from build123d import *

# Parameters (mm, degrees)
BOSS_EXTRUDE1_DEPTH = 7.5
SKETCH2_W           = 10
SKETCH2_H           = 10
BOSS_EXTRUDE2_DEPTH = 12


with BuildPart() as part:
    # Sketch1 → Boss-Extrude1 (new, symmetric)
    with BuildSketch(Plane(origin=(0, 0, 0), x_dir=(1, 0, 0), z_dir=(0, 1, 0))):
        Polygon((25, 107.5), (35, 107.5), (35, -117.5), (-35, -117.5), (-35, 107.5), (-25, 107.5), (-25, -107.5), (25, -107.5), align=None)
    extrude(amount=BOSS_EXTRUDE1_DEPTH, both=True)

    # Sketch2 → Boss-Extrude2 (add)
    with BuildSketch(Plane(origin=(0, 0, -107.5), x_dir=(-1, 0, 0), z_dir=(0, 0, -1))):
        with Locations((-30, 12.5)):
            Rectangle(SKETCH2_W, SKETCH2_H)
        Polygon((-35, 21.5), (-35, 17.5), (-25, 17.5), (25, 17.5), (35, 17.5), (35, 21.5), align=None)
        with Locations((30, 12.5)):
            Rectangle(SKETCH2_W, SKETCH2_H)
    extrude(amount=-BOSS_EXTRUDE2_DEPTH)


solid = part.part
Part model, mm, in its own coordinate system. A direction names the side the tool comes from. Coordinates: 2 decimals unless noted, no trailing zeros. Write each loop counter-clockwise with the first axis right and the second up, starting at its lowest first coordinate (ties: lowest second). Pieces come first, ordered by that corner, then holes. Notation, with made-up numbers: (-27.5, -5) - (4.5, -5) arc R31 cw to (4.5, 33) - close; hole circle Ø3 at (70.5, 44). An arc over 180 degrees is marked (long way). Put each result on its own line as item: value.
1. Band-saw the part on B-B (z = -49). Write the cut outline in (x, y), then the cut area to 3 significant figures.
Final values:
outline: (-35, -7.5) - (-25, -7.5) - (-25, 7.5) - (-35, 7.5) - close; (25, -7.5) - (35, -7.5) - (35, 7.5) - (25, 7.5) - close
area: 300 mm²
2. Band-saw the part on C-C (y = -3.5). Write the cut outline in (x, z), then the cut area to 3 significant figures.
Final values:
outline: (-35, -107.5) - (-25, -107.5) - (-25, 107.5) - (25, 107.5) - (25, -107.5) - (35, -107.5) - (35, 117.5) - (-35, 117.5) - close
area: 5,000 mm²
3. Two-plate mould, pull along X, no slides. Class faces 1 (the flat face through (0, 21.5, -102)), 2 (the flat face through (35, 1, 3)), 3 (the flat face through (0, 17.5, -102)): +X half, -X half, draft (parallel to the pull), parting line (faces both ways), or undercut.
Final values:
face 1: draft
face 2: +X half
face 3: undercut
4. Band-saw the part on A-A (x = -19). Write the cut outline in (y, z).
Final values:
outline: (-7.5, 107.5) - (7.5, 107.5) - (7.5, 117.5) - (-7.5, 117.5) - close; (17.5, -107.5) - (21.5, -107.5) - (21.5, -95.5) - (17.5, -95.5) - close
5. Band-saw the part on D-D (x = 30). Write the cut outline in (y, z).
Final values:
outline: (-7.5, -107.5) - (21.5, -107.5) - (21.5, -95.5) - (7.5, -95.5) - (7.5, 117.5) - (-7.5, 117.5) - close
6. 3-axis set-ups, long thin cutter, end or side, ignore diameter. For faces 4 (the flat face through (0, 0, 107.5)), 5 (the flat face through (0, 0, 117.5)), 6 (the flat face through (-26, 7.5, 18)), 7 (the flat face through (25, -1, -2)): which of +Z, -Z, +X, -X, +Y, -Y reach the whole face in a straight line?
Final values:
face 4: -Z, +Y, -Y
face 5: +Z, +X, -X, +Y, -Y
face 6: +Z, +X, -X, +Y
face 7: -Z, -Y
7. Probe line 1 along X through (y, z) = (6.25, -75.5); line 2 along Z through (x, y) = (17, 6); line 3 along Z through (x, y) = (3, 20). List the from-to ranges inside material, lowest first. Write a range as [from, to].
Final values:
line 1: x = [-35, -25], [25, 35]
line 2: z = [107.5, 117.5]
line 3: z = [-107.5, -95.5]
8. Flat gauge pins, fed straight in: pin 1 Ø4.5 at (x, y) = (-8, 2) entering from -Z; pin 2 Ø11 at (x, y) = (-11, 16.5) entering from +Z; pin 3 Ø13 at (x, z) = (11.5, -101.5) entering from -Y; pin 4 Ø2 at (x, y) = (-10, 10) entering from -Z. Where does each tip first touch, or does it go through?
Final values:
pin 1: stops at z = 107.5
pin 2: stops at z = -95.5
pin 3: stops at y = 17.5
pin 4: passes through
